Can you work these out from the model? Positions are in its coordinate system, mm. Face numbers are marked on the shaded views. Give positions to 0.01 mm unless a question says otherwise; leave off trailing zeros. Loops run counter-clockwise (first coordinate to the right, second up) from the corner with the lowest first, then second, coordinate; pieces in that order, holes last.
from build123d import *

# Parameters (mm, degrees)
F0_R     = 3.5687
F1_DEPTH = 12.7
F3_SIZE  = 0.79375


# Not quite as in the source:
# - a fillet or chamfer that OpenCascade refuses, or shapes differently, is made with other operations: its cross-section is extruded or revolved along the edge and cut away or added


with BuildPart() as f1:
    # F0 (on Top) → F1 (new body)
    with BuildSketch(Plane.XY):
        with BuildLine():
            Line((0, 10.31875), (0, 25.4))
            ThreePointArc((0, 25.4), (-25.4, 0), (0, -25.4))
            Line((0, -25.4), (0, -10.31875))
            ThreePointArc((0, -10.31875), (-10.31875, 0), (0, 10.31875))
        make_face()
        with BuildLine():
            ThreePointArc((0, 25.4), (17.9605122421, 17.9605122421), (25.4, 0))
            ThreePointArc((25.4, 0), (17.9605122421, -17.9605122421), (0, -25.4))
            Line((0, -25.4), (63.5, -25.4))
            Line((63.5, -25.4), (63.5, 25.4))
            Line((63.5, 25.4), (0, 25.4))
        make_face()
        with Locations((50.8, -12.7)):
            Circle(F0_R, mode=Mode.SUBTRACT)
        with Locations((50.8, 12.7)):
            Circle(F0_R, mode=Mode.SUBTRACT)
        with BuildLine():
            ThreePointArc((0, -25.4), (17.9605122421, -17.9605122421), (25.4, 0))
            ThreePointArc((25.4, 0), (17.9605122421, 17.9605122421), (0, 25.4))
            Line((0, 25.4), (0, 10.31875))
            ThreePointArc((0, 10.31875), (7.2964580984, 7.2964580984), (10.31875, 0))
            ThreePointArc((10.31875, 0), (7.2964580984, -7.2964580984), (0, -10.31875))
            Line((0, -10.31875), (0, -25.4))
        make_face()
    extrude(amount=F1_DEPTH)

    # F2: chamfer of 1.5875 on 2 edges, made by hand

    # F2_s1 → F2_t2 (revolve, cut)
    with BuildSketch(Plane.YZ):
        Polygon((10.31875, 1.5875), (11.90625, 0), (10.31875, 0), align=None)
    revolve(axis=Axis((0, 0, 0), (0, 0, -1)), mode=Mode.SUBTRACT)

    # F2_s3 → F2_t4 (revolve, cut)
    with BuildSketch(Plane.YZ):
        Polygon((10.31875, 11.1125), (11.90625, 12.7), (10.31875, 12.7), align=None)
    revolve(axis=Axis((0, 0, 12.7), (0, 0, -1)), mode=Mode.SUBTRACT)

    # F3
    f3_edges = [f1.edges().sort_by_distance(p)[0] for p in [
        (47.2313, -12.7, 0),
        (47.2313, 12.7, 0),
        (47.2313, -12.7, 12.7),
        (47.2313, 12.7, 12.7),
    ]]
    chamfer(f3_edges, length=F3_SIZE)


solid = f1.part
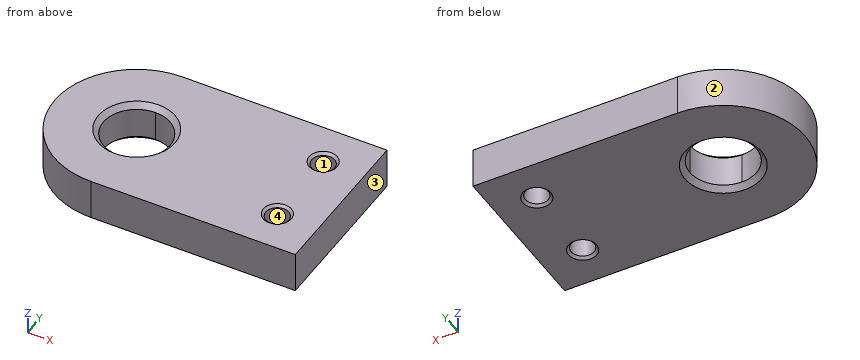
(1) Will these pins go through, and if not, where does the flat tip stop? P1, Ø4.5, axis at x = 50.8, y = -12.7, coming from the -Z side; P2, Ø8, axis at x = 50.8, y = 12.7, coming from the +Z side; P3, Ø6, axis at y = -0.5, z = 5.5, coming from the -X side; P4, Ø2, axis at y = 8.5, z = 6.5, coming from the -X side.
Returned:
P1: passes through
P2: stops at z = 12.34
P3: stops at x = -25.4
P4: stops at x = -24.27
(2) Please list where these lines run through material, in increasing order: probe 1 along Y at (x, z) = (50.8, 6.5); probe 2 along Y at (x, z) = (4, 10.5); probe 3 along X at (y, z) = (-15, 2.75).
Returned:
probe 1: y = -25.4 to -16.27, -9.13 to 9.13, 16.27 to 25.4
probe 2: y = -25.4 to -9.51, 9.51 to 25.4
probe 3: x = -20.5 to 48.07, 53.53 to 63.5
(3) Suppose I cut it at B-B on x = 50.8. List the corners of the cut face in (y, z) for me, plus the area to 3 significant figures.
Returned:
outline: (-25.4, 0) - (-17.06, 0) - (-16.27, 0.79) - (-16.27, 11.91) - (-17.06, 12.7) - (-25.4, 12.7) - close; (-9.13, 0.79) - (-8.34, 0) - (8.34, 0) - (9.13, 0.79) - (9.13, 11.91) - (8.34, 12.7) - (-8.34, 12.7) - (-9.13, 11.91) - close; (16.27, 0.79) - (17.06, 0) - (25.4, 0) - (25.4, 12.7) - (17.06, 12.7) - (16.27, 11.91) - close
area: 461 mm2
(4) Suppose I cut it at C-C on y = -20. List the corners of the cut face in (x, z) for me.
Returned:
outline: (-15.66, 0) - (63.5, 0) - (63.5, 12.7) - (-15.66, 12.7) - close
(5) Suppose I cut it at A-A on z = 8. List the corners of the cut face in (x, y) for me.
Returned:
outline: (0, -25.4) - (63.5, -25.4) - (63.5, 25.4) - (0, 25.4) arc R25.4 ccw to start; hole circle Ø20.64 at (0, 0); hole circle Ø7.14 at (50.8, -12.7); hole circle Ø7.14 at (50.8, 12.7)
(6) Thinking about a two-plate mould opening in Y: for the marked faces 1, 2, 3 and 4, which applies, pulls with the +Y half, pulls with the -Y half, needs draft (parallel to the pull), parting line crosses it, or undercut?
Returned:
face 1: undercut
face 2: parting line crosses it
face 3: needs draft
face 4: undercut
